Design review of the part built by this model. Coordinates are the model's own, in mm. Coordinates: 2 decimals unless noted, no trailing zeros. Write each loop counter-clockwise with the first axis right and the second up, starting at its lowest first coordinate (ties: lowest second). Pieces come first, ordered by that corner, then holes. Notation, with made-up numbers: (67, 22) - (89, 22) arc R20 cw to (89, 36) - close; hole circle Ø6 at (74, -3.5). An arc over 180 degrees is marked (long way). Answer as a JSON object with one key per item and string values.
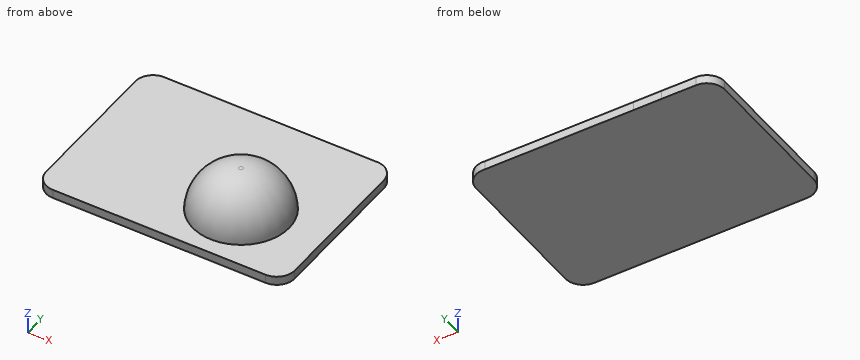
```python
from build123d import *

# Parameters (mm, degrees)
F0_R     = 34.544
F1_DEPTH = 38.1
F2_R     = 33.02
F4_DEPTH = 6.35


# Not quite as in the source:
# - the program builds the solid bodies; features that only make, move or delete a surface that nothing else refers to are left out


with BuildPart() as f1:
    # F0 (on Top) → F1 (new body)
    with BuildSketch(Plane.XY):
        with Locations((29.9727506936, -18.0700458586)):
            Circle(F0_R)
    extrude(amount=F1_DEPTH)

    # F2
    f2_edges = [f1.edges().sort_by_distance(p)[0] for p in [
        (-4.571249, -18.070046, 38.1),
    ]]
    fillet(f2_edges, radius=F2_R)

    # F0 (on Top) → F4 (join)
    with BuildSketch(Plane.XY):
        with BuildLine():
            Line((-76.2, -63.5), (76.2, -63.5))
            ThreePointArc((76.2, -63.5), (85.1802561211, -59.7802561211), (88.9, -50.8))
            Line((88.9, -50.8), (88.9, 50.8837117301))
            ThreePointArc((88.9, 50.8837117301), (84.6499025139, 60.364700471), (74.7442287394, 63.500000013))
            Line((74.7442287394, 63.500000013), (-31.496, 63.500000013))
            Line((-31.496, 63.500000013), (-51.816, 63.5))
            Line((-51.816, 63.5), (-76.2, 63.5))
            ThreePointArc((-76.2, 63.5), (-85.1802561211, 59.7802561211), (-88.9, 50.8))
            Line((-88.9, 50.8), (-88.9, -50.8))
            ThreePointArc((-88.9, -50.8), (-85.1802561211, -59.7802561211), (-76.2, -63.5))
        make_face()
        with Locations((29.9727506936, -18.0700458586)):
            Circle(F0_R, mode=Mode.SUBTRACT)
    extrude(amount=F4_DEPTH)


solid = f1.part
```
(1) For pin 1 (2 mm diameter, centred on x = 61.5, y = -45.5, fed in from +Z); pin 2 (6 mm diameter, centred on x = 45, y = -37.5, fed in from +Z); pin 3 (5 mm diameter, centred on x = 29, z = 4, fed in from +Y); pin 4 (2 mm diameter, centred on x = 69, z = 8, fed in from +Y), all flat-tipped, find the tip position at first contact; note any pin that passes through.
Solved:
{"pin 1": "stops at z = 6.35", "pin 2": "stops at z = 31.32", "pin 3": "stops at y = 63.5", "pin 4": "passes through"}
(2) Take a section at B-B, the plane y = 27. Write out the cut boundary in (x, z), and give its area (3 significant figures).
Solved:
{"outline": "(-88.9, 0) - (88.9, 0) - (88.9, 6.35) - (-88.9, 6.35) - close", "area": "1,130 mm^2"}
(3) Take a section at A-A, the plane x = -9.5. Write out the cut boundary in (y, z), and give its area (3 significant figures).
Solved:
{"outline": "(-63.5, 0) - (63.5, 0) - (63.5, 6.35) - (-63.5, 6.35) - close", "area": "806 mm^2"}
(4) To check wall thickness, follow line 1 (Z direction, x = 48.5, y = 39.5); line 2 (Y direction, x = 72.5, z = 2.5); line 3 (X direction, y = -4, z = 32). State the ranges of each line that lie inside material, in increasing order. Write a range as from..to.
Solved:
{"line 1": "z = 0..6.35", "line 2": "y = -63.5..63.5", "line 3": "x = 14.86..45.08"}
